For this review, use the dimensioned drawing (mm, ordinates from the lowest corner) and the shaded views. A direction names the side the tool comes from. Coordinates: 2 decimals unless noted, no trailing zeros. Order: outer loops, then holes, each group sorted by start corner. A loop starts at its lowest first (then second) coordinate and runs counter-clockwise, first axis right, second up. Notation, with made-up numbers: M -3.75,74.5 L 32.25,74.5 A11 ccw 32.25,86.5 Z; hole C 34,31.5 d5. An arc over 180 degrees is marked long. Use CSV: the item, a comma, the result in double quotes.
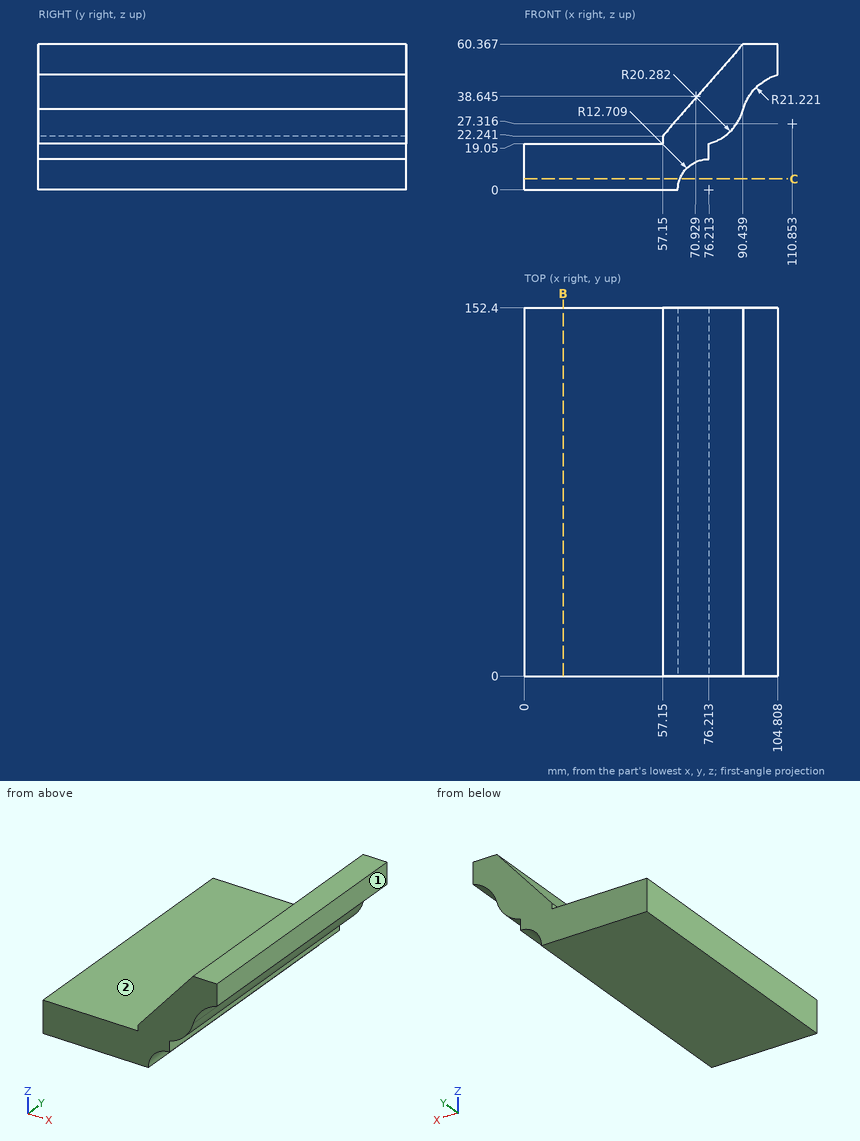
Item 1: To check wall thickness, follow line 1 along Z through (x, y) = (4.5, 106.5); line 2 along Z through (x, y) = (63, 39); line 3 along X through (y, z) = (61, 39.5). State the ranges of each line that lie inside material, in increasing order. Write a range as [from, to].
Solutions:
line 1,"[0, 19.05]"
line 2,"[0, 28.94]"
line 3,"[72.22, 93.48]"
Item 2: Clearance check with flat-ended pins moving along their axes: pin 1 Ø12 at (y, z) = (46, 50.5) entering from -X (1 decimal); pin 2 Ø17 at (x, y) = (22, 49.5) entering from +Z; pin 3 Ø1.5 at (y, z) = (17.5, 30.5) entering from -X (1 decimal). State where each tip first meets the part, or that it passes through.
Solutions:
pin 1,"x = 76.6"
pin 2,"z = 19.05"
pin 3,"x = 63.7"
Item 3: Add section B-B on x = 16. State the section outline as (y, z) points.
Solutions:
outline,"M 0,0 L 152.4,0 L 152.4,19.05 L 0,19.05 Z"
Item 4: Add section C-C on z = 4.5. State the section outline as (x, y) points.
Solutions:
outline,"M 0,0 L 64.33,0 L 64.33,152.4 L 0,152.4 Z"
Item 5: For the marked faces 1 and 2, list the 3-axis set-ups (+Z, -Z, +X, -X, +Y, -Y) from which the entire face can be reached by the end or side of a thin tool; tool diameter is ignored.
Solutions:
face 1,"+Z, -Z, +X, +Y, -Y"
face 2,"+Z, -X, +Y, -Y"
